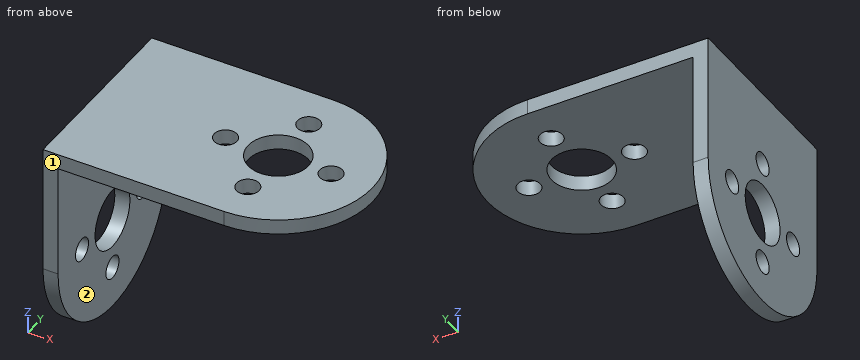
Autodesk Inventor part; units mm, degrees
ref_plane "YZ Plane" through (0, 0, 0) normal (1, 0, 0) x (0, 1, 0)
ref_plane "XZ Plane" through (0, 0, 0) normal (0, 1, 0) x (-1, 0, 0)
ref_plane "XY Plane" through (0, 0, 0) normal (0, 0, 1) x (1, 0, 0)
sketch "Sketch1" plane through (0, 0, 0) normal (0, 0, 1) x (1, 0, 0)
  line L0 (0, 0) -> (24, 0)
  line L1 (24, 25) -> (0, 25)
  line L2 (0, 25) -> (0, 0)
  arc A0 (24, 0) -> (24, 25) centre (24, 12.5) ccw
  circle A1 centre (24, 12.5) radius 4
  circle A2 centre (24, 12.5) radius 7
  circle A3 centre (24, 19.5) radius 1.5
  circle A4 centre (17, 12.5) radius 1.5
  circle A5 centre (24, 5.5) radius 1.5
  circle A6 centre (31, 12.5) radius 1.5
  line L3 (24, 0) -> (24, 16.5)
  line L4 (24, 19.5) -> (24, 21)
  line L5 (0, 25) -> (2, 25)
  line L6 (2, 25) -> (2, 0)
  line L7 (2, 0) -> (0, 0)
  line L8 (0, 0) -> (0, 25)
  dimension "d2" = 8
  dimension "d3" = 14
  dimension "d4" = 3
  dimension "d0" = 24
  dimension "d1" = 25
  dimension "d7" = 360
  dimension "d11" = 2
extrude "Extrusion1" add sketch "Sketch1" along normal blind 2 contours L2 L1 L6 L0 | L6 L1 A0 L0 | A2 A4 A3 A6 A5
extrude "Extrusion2" add sketch "Sketch1" against normal blind 1 contours L2 L1 L6 L0
sketch "Sketch2" plane through (2, 0, 0) normal (1, 0, 0) x (0, 0, -1)
  line L0 (0, 25) -> (0, 0)
  line L1 (0, 25) -> (15, 25)
  line L2 (15, 25) -> (15, 0)
  line L3 (15, 0) -> (0, 0)
  line L4 (0, 0) -> (0, 25)
  circle A0 centre (15, 12.5) radius 12.5
  circle A1 centre (15, 12.5) radius 4
  circle A2 centre (15, 12.5) radius 7
  circle A3 centre (15, 19.5) radius 1.5
  circle A4 centre (8, 12.5) radius 1.5
  circle A5 centre (15, 5.5) radius 1.5
  circle A6 centre (22, 12.5) radius 1.5
  point P0 (15, 0)
  dimension "d17" = 14
  dimension "d14" = 15
  dimension "d15" = 25
  dimension "d16" = 8
  dimension "d18" = 3
  dimension "d21" = 360
extrude "Extrusion3" add sketch "Sketch2" against normal blind 2 contours L1 A0 L3 L0 | A0 L2 A5 A2 A6 A3 | L2 A3 A2 A4 A5 A0 | A3 L2 A1 A5 A2 A4 | A3 A2 A6 A5 L2 A1
properties part number "Bracket ANGULO"
Read the model definition and answer for the solid it produces. Units are mm, in the model's axes. Face numbers are marked on the shaded views. A direction names the side the tool comes from. Coordinates: 2 decimals unless noted, no trailing zeros. Write each loop counter-clockwise with the first axis right and the second up, starting at its lowest first coordinate (ties: lowest second). Pieces come first, ordered by that corner, then holes. Notation, with made-up numbers: (36, -7.75) -> (44, -7.75) arc R27 cw to (44, 22.25) -> close; hole circle Ø11 at (-34, 38.5). An arc over 180 degrees is marked (long way). Write item = value, one per line.
(1) Given pin 1 Ø10.5 at (x, y) = (24, 12.5) entering from -Z; pin 2 Ø2.5 at (y, z) = (19.5, -15) entering from +X; pin 3 Ø8 at (y, z) = (17, -18) entering from +X, each flat-ended and moving along its own axis, determine where each tip first touches the part or whether it passes through.
From the geometry:
pin_1 = 0
pin_2 = through
pin_3 = 2
(2) Section D-D on z = -16 is taken. Write down the section's boundary in (x, y).
From the geometry:
outline = (0, 0.04) -> (2, 0.04) -> (2, 4.38) -> (0, 4.38) -> close; (0, 6.62) -> (2, 6.62) -> (2, 8.63) -> (0, 8.63) -> close; (0, 16.37) -> (2, 16.37) -> (2, 18.38) -> (0, 18.38) -> close; (0, 20.62) -> (2, 20.62) -> (2, 24.96) -> (0, 24.96) -> close
(3) Section C-C on y = 20 is taken. Write down the section's boundary in (x, z).
From the geometry:
outline = (0, -25) -> (2, -25) -> (2, -16.41) -> (0, -16.41) -> close; (0, -13.59) -> (2, -13.59) -> (2, 0) -> (22.59, 0) -> (22.59, 2) -> (0, 2) -> close; (25.41, 0) -> (34, 0) -> (34, 2) -> (25.41, 2) -> close
(4) Straight lines are drawn through the part: L1, parallel to X at y = 12.5, z = 1.2; L2, parallel to Y at x = 24, z = 0.8; L3, parallel to Z at x = 1.15, y = 12.5. For each, find the intervals that lie inside material, in ascending order. Write a range as from..to.
From the geometry:
L1 = 0..15.5, 18.5..20, 28..29.5, 32.5..36.5
L2 = 0..4, 7..8.5, 16.5..18, 21..25
L3 = -27.5..-23.5, -20.5..-19, -11..-9.5, -6.5..2
(5) Section A-A on z = -8 is taken. Write down the section's boundary in (x, y).
From the geometry:
outline = (0, 0) -> (2, 0) -> (2, 11) -> (0, 11) -> close; (0, 14) -> (2, 14) -> (2, 25) -> (0, 25) -> close
(6) Which of the six approach directions +Z, -Z, +X, -X, +Y, -Y give full straight-line access (tool end or side, diameter ignored) to the marked faces 1 and 2?
From the geometry:
face_1 = +Z, -Z, +X, -X, -Y
face_2 = -Z, +X, +Y, -Y
(7) Section B-B on x = 17 is taken. Write down the section's boundary in (y, z), plus the area to 3 significant figures.
From the geometry:
outline = (0, 0) -> (11, 0) -> (11, 2) -> (0, 2) -> close; (14, 0) -> (25, 0) -> (25, 2) -> (14, 2) -> close
area = 44.0 mm2
